Source: CAD feature listing. Evaluate the final solid. Frame: model axes, mm. Give positions to 0.01 mm unless a question says otherwise; leave off trailing zeros. Loops run counter-clockwise (first coordinate to the right, second up) from the corner with the lowest first, then second, coordinate; pieces in that order, holes last.
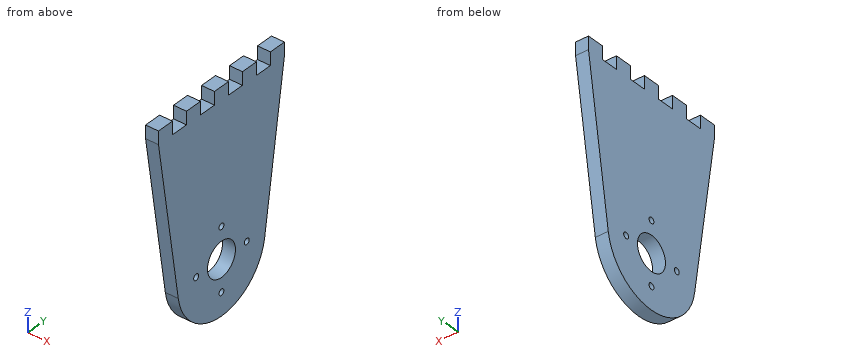
```python
from build123d import *

# Parameters (mm, degrees)
SKETCH1_R           = 4
SKETCH1_R_2         = 0.7
BOSS_EXTRUDE1_DEPTH = 3


with BuildPart() as part:
    # Sketch1 → Boss-Extrude1 (new body)
    with BuildSketch(Plane(origin=(0, 0, 0), x_dir=(0, 0, -1), z_dir=(1, 0, 0))):
        with BuildLine():
            Line((-38, 18), (-35, 18))
            Line((-35, 18), (1.890350117, 12.356236338))
            ThreePointArc((1.890350117, 12.356236338), (12.5, 0), (1.890350117, -12.356236338))
            Line((1.890350117, -12.356236338), (-35, -18))
            Line((-35, -18), (-38, -18))
            Line((-38, -18), (-38, -14))
            Line((-38, -14), (-35, -14))
            Line((-35, -14), (-35, -10))
            Line((-35, -10), (-38, -10))
            Line((-38, -10), (-38, -6))
            Line((-38, -6), (-35, -6))
            Line((-35, -6), (-35, -2))
            Line((-35, -2), (-38, -2))
            Line((-38, -2), (-38, 2))
            Line((-38, 2), (-35, 2))
            Line((-35, 2), (-35, 6))
            Line((-35, 6), (-38, 6))
            Line((-38, 6), (-38, 10))
            Line((-38, 10), (-35, 10))
            Line((-35, 10), (-35, 14))
            Line((-35, 14), (-38, 14))
            Line((-38, 14), (-38, 18))
        make_face()
        Circle(SKETCH1_R, mode=Mode.SUBTRACT)
        with Locations((-7.24, 0)):
            Circle(SKETCH1_R_2, mode=Mode.SUBTRACT)
        with Locations((0, 7.24)):
            Circle(SKETCH1_R_2, mode=Mode.SUBTRACT)
        with Locations((7.24, 0)):
            Circle(SKETCH1_R_2, mode=Mode.SUBTRACT)
        with Locations((0, -7.24)):
            Circle(SKETCH1_R_2, mode=Mode.SUBTRACT)
    extrude(amount=BOSS_EXTRUDE1_DEPTH)


solid = part.part
```
(1) Section B-B, the plane z = 3.5. Return the cut outline in (x, y).
A:
outline: (0, -13.18) - (3, -13.18) - (3, -1.94) - (0, -1.94) - close; (0, 1.94) - (3, 1.94) - (3, 13.18) - (0, 13.18) - close
(2) First-contact query: pin 1 (1.8 mm diameter, centred on y = 0, z = 7.24, fed in from +X); pin 2 (1.5 mm diameter, centred on x = 1, y = -3, fed in from +Z). Flat tips, straight axial feed; report the tip coordinate or a pass-through.
A:
pin 1: stops at x = 3
pin 2: stops at z = 35
(3) Section A-A, the plane y = 0. Return the cut outline in (x, z), then the cut area to 3 significant figures.
A:
outline: (0, -12.5) - (3, -12.5) - (3, -7.94) - (0, -7.94) - close; (0, -6.54) - (3, -6.54) - (3, -4) - (0, -4) - close; (0, 4) - (3, 4) - (3, 6.54) - (0, 6.54) - close; (0, 7.94) - (3, 7.94) - (3, 38) - (0, 38) - close
area: 119 mm2
(4) Section C-C, the plane x = 1.45. Return the cut outline in (y, z), then the cut area to 3 significant figures.
A:
outline: (-18, 35) - (-12.36, -1.89) arc R12.5 ccw to (12.36, -1.89) - (18, 35) - (18, 38) - (14, 38) - (14, 35) - (10, 35) - (10, 38) - (6, 38) - (6, 35) - (2, 35) - (2, 38) - (-2, 38) - (-2, 35) - (-6, 35) - (-6, 38) - (-10, 38) - (-10, 35) - (-14, 35) - (-14, 38) - (-18, 38) - close; hole circle Ø1.4 at (-7.24, 0); hole circle Ø8 at (0, 0); hole circle Ø1.4 at (0, -7.24); hole circle Ø1.4 at (0, 7.24); hole circle Ø1.4 at (7.24, 0)
area: 1,320 mm2
(5) Section D-D, the plane y = 7.24. Return the cut outline in (x, z), then the cut area to 3 significant figures.
A:
outline: (0, -10.19) - (3, -10.19) - (3, -0.7) - (0, -0.7) - close; (0, 0.7) - (3, 0.7) - (3, 38) - (0, 38) - close
area: 140 mm2
(6) Ray query, line 1 along Y through (x, z) = (0.6, 0); line 2 along Y through (x, z) = (1.25, 7.24); line 3 along Y through (x, z) = (0.2, -2.5). Return the intervals inside material, ascending.
A:
line 1: y = -12.65 to -7.94, -6.54 to -4, 4 to 6.54, 7.94 to 12.65
line 2: y = -13.75 to -0.7, 0.7 to 13.75
line 3: y = -12.25 to -3.12, 3.12 to 12.25
